Geometry: see drawing. Coordinates: mm, zero at the bounding-box minimum. Round coordinates to 2 decimals unless told otherwise and drop trailing zeros. Order: outer loops, then holes, each group sorted by start corner. A loop starts at its lowest first (then second) coordinate and runs counter-clockwise, first axis right, second up. Notation, with made-up numbers: (81.5, 89) -> (127.5, 89) arc R3 cw to (127.5, 94) -> close; hole circle Ø10 at (41.25, 68.25). An arc over 180 degrees is marked (long way). Use a Markdown table: item, result.
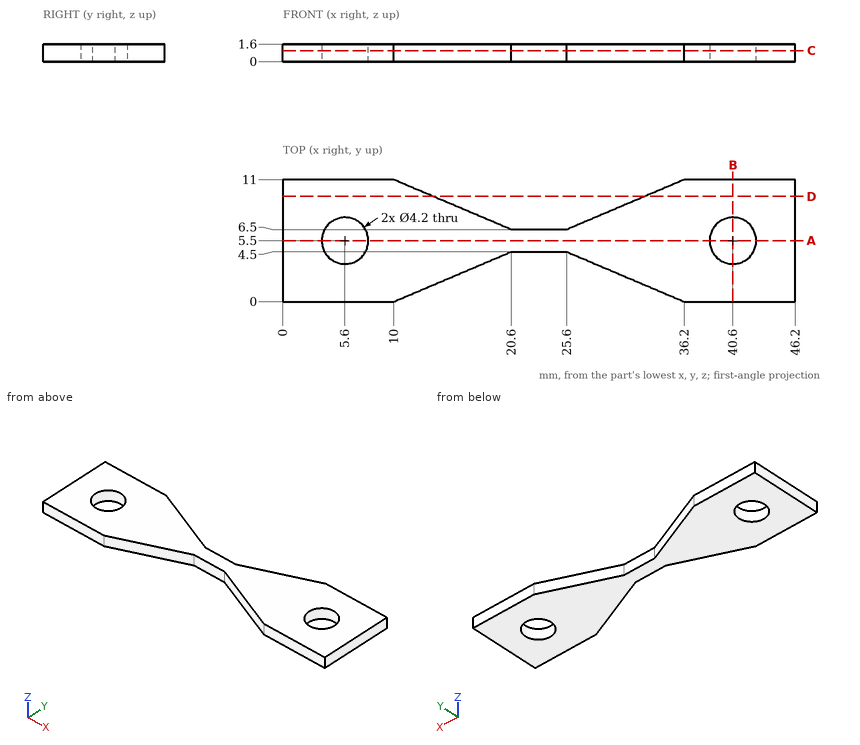
1) Cut plane D-D on y = 9.5. Return loops of the section in (x, z).
Answer key:
| item | result |
|---|---|
| outline | (0, 0) -> (13.53, 0) -> (13.53, 1.6) -> (0, 1.6) -> close; (32.67, 0) -> (46.2, 0) -> (46.2, 1.6) -> (32.67, 1.6) -> close |
2) Ray query, probe 1 along Y at (x, z) = (5.6, 0.95); probe 2 along X at (y, z) = (6, 0.75); probe 3 along X at (y, z) = (1.5, 1.05). Return the intervals inside material, ascending.
Answer key:
| item | result |
|---|---|
| probe 1 | y = 0 to 3.4, 7.6 to 11 |
| probe 2 | x = 0 to 3.56, 7.64 to 38.56, 42.64 to 46.2 |
| probe 3 | x = 0 to 13.53, 32.67 to 46.2 |
3) Cut plane B-B on x = 40.6. Return loops of the section in (y, z), and give its area (3 significant figures).
Answer key:
| item | result |
|---|---|
| outline | (0, 0) -> (3.4, 0) -> (3.4, 1.6) -> (0, 1.6) -> close; (7.6, 0) -> (11, 0) -> (11, 1.6) -> (7.6, 1.6) -> close |
| area | 10.9 mm^2 |
4) Cut plane A-A on y = 5.5. Return loops of the section in (x, z), and give its area (3 significant figures).
Answer key:
| item | result |
|---|---|
| outline | (0, 0) -> (3.5, 0) -> (3.5, 1.6) -> (0, 1.6) -> close; (7.7, 0) -> (38.5, 0) -> (38.5, 1.6) -> (7.7, 1.6) -> close; (42.7, 0) -> (46.2, 0) -> (46.2, 1.6) -> (42.7, 1.6) -> close |
| area | 60.5 mm^2 |
5) Contact query for flat-ended pins moving along their axis: P1, Ø0.8, axis at x = 23, z = 1, coming from the -Y side; P2, Ø0.8, axis at x = 23, z = 0.5, coming from the +Y side. Output: stop coordinate, or through.
Answer key:
| item | result |
|---|---|
| P1 | stops at y = 4.5 |
| P2 | stops at y = 6.5 |
6) Cut plane C-C on z = 1. Return loops of the section in (x, y).
Answer key:
| item | result |
|---|---|
| outline | (0, 0) -> (10, 0) -> (20.6, 4.5) -> (25.6, 4.5) -> (36.2, 0) -> (46.2, 0) -> (46.2, 11) -> (36.2, 11) -> (25.6, 6.5) -> (20.6, 6.5) -> (10, 11) -> (0, 11) -> close; hole circle Ø4.2 at (5.6, 5.5); hole circle Ø4.2 at (40.6, 5.5) |
